Geometry check sheet. Reference: the model listing, model coordinates, mm. Round coordinates to 2 decimals unless told otherwise and drop trailing zeros. Write each loop counter-clockwise with the first axis right and the second up, starting at its lowest first coordinate (ties: lowest second). Pieces come first, ordered by that corner, then holes. Notation, with made-up numbers: M 80.5,-29.5 L 108.5,-29.5 A13 ccw 108.5,-14.5 Z; hole C 28,45 d3. An arc over 180 degrees is marked long. One line per item, written item: value. Start each with the question number.
1. Scan lines: probe 1 along X at (y, z) = (41, 3.05); probe 2 along Y at (x, z) = (2, 2.2). Record each from-to range of solid material in increasing order. Write a range as [from, to].
2. Section check A-A (y = -26). Record the boundary of the cut face in (x, z) (3 decimals), and give its area (3 significant figures).
3. Section check C-C (z = 2.4). Record the boundary of the cut face in (x, y).
4. Section check B-B (x = 9). Record the boundary of the cut face in (y, z) (3 decimals).
from build123d import *

# Parameters (mm, degrees)
SKETCH1_W           = 508.2032
SKETCH1_H           = 131.97205
SKETCH1_W_2         = 393.4968
SKETCH1_H_2         = 101.4476
BOSS_EXTRUDE1_DEPTH = 3.175


with BuildPart() as part:
    # Sketch1 → Boss-Extrude1 (new body)
    with BuildSketch(Plane.XY):
        Rectangle(SKETCH1_W, SKETCH1_H)
        with Locations((-6.35, -0.0254)):
            Rectangle(SKETCH1_W_2, SKETCH1_H_2, mode=Mode.SUBTRACT)
    extrude(amount=BOSS_EXTRUDE1_DEPTH)


solid = part.part
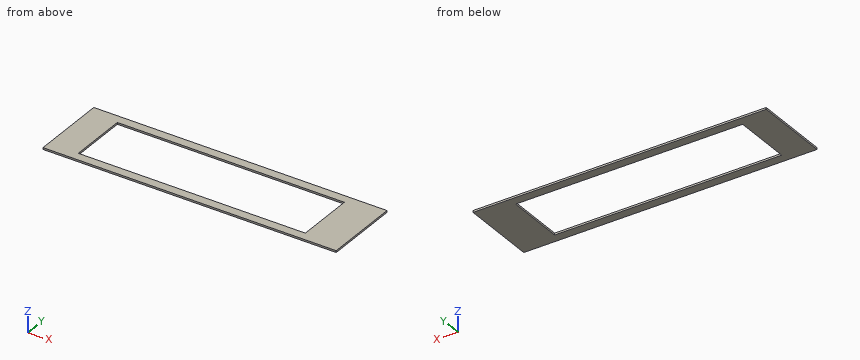
Result sheet:
1. probe 1: x = [-254.1, -203.1], [190.4, 254.1]
1. probe 2: y = [-65.99, -50.75], [50.7, 65.99]
2. outline: M -254.102,0 L -203.098,0 L -203.098,3.175 L -254.102,3.175 Z; M 190.398,0 L 254.102,0 L 254.102,3.175 L 190.398,3.175 Z
2. area: 364 mm2
3. outline: M -254.1,-65.99 L 254.1,-65.99 L 254.1,65.99 L -254.1,65.99 Z; hole M -203.1,-50.75 L 190.4,-50.75 L 190.4,50.7 L -203.1,50.7 Z
4. outline: M -65.986,0 L -50.749,0 L -50.749,3.175 L -65.986,3.175 Z; M 50.698,0 L 65.986,0 L 65.986,3.175 L 50.698,3.175 Z
